from build123d import *

# Parameters (mm, degrees)
SKETCH1_R           = 8
SKETCH1_R_2         = 1.75
BOSS_EXTRUDE1_DEPTH = 6.35
FILLET1_R           = 10


with BuildPart() as part:
    # Sketch1 → Boss-Extrude1 (new body)
    with BuildSketch(Plane(origin=(0, 0, 0), x_dir=(1, 0, 0), z_dir=(0, 1, 0))):
        Polygon((0, 44.633081493), (33.8, 0), (88, 0), (88, 300), (33.8, 300), (0, 280.510901235), align=None)
        with Locations(Location((13, 49, 0), (0, 0, 270))):
            Circle(SKETCH1_R, mode=Mode.SUBTRACT)
        with Locations(Location((38.8, 25, 0), (0, 0, 270))):
            Circle(SKETCH1_R_2, mode=Mode.SUBTRACT)
        with Locations(Location((38.8, 69.2, 0), (0, 0, 270))):
            Circle(SKETCH1_R_2, mode=Mode.SUBTRACT)
        with Locations(Location((18, 84.2, 0), (0, 0, 270))):
            Circle(SKETCH1_R_2, mode=Mode.SUBTRACT)
        with Locations(Location((45, 5, 0), (0, 0, 270))):
            Circle(SKETCH1_R_2, mode=Mode.SUBTRACT)
        with Locations(Location((76.8, 5, 0), (0, 0, 270))):
            Circle(SKETCH1_R_2, mode=Mode.SUBTRACT)
        with Locations(Location((83, 25, 0), (0, 0, 270))):
            Circle(SKETCH1_R_2, mode=Mode.SUBTRACT)
        with Locations(Location((83, 69.2, 0), (0, 0, 270))):
            Circle(SKETCH1_R_2, mode=Mode.SUBTRACT)
        with Locations(Location((70, 84.2, 0), (0, 0, 270))):
            Circle(SKETCH1_R_2, mode=Mode.SUBTRACT)
        with Locations(Location((18, 211.2, 0), (0, 0, 270))):
            Circle(SKETCH1_R_2, mode=Mode.SUBTRACT)
        with Locations(Location((4, 226.2, 0), (0, 0, 270))):
            Circle(SKETCH1_R_2, mode=Mode.SUBTRACT)
        with Locations(Location((4, 278.2, 0), (0, 0, 270))):
            Circle(SKETCH1_R_2, mode=Mode.SUBTRACT)
        with Locations(Location((70, 211.2, 0), (0, 0, 270))):
            Circle(SKETCH1_R_2, mode=Mode.SUBTRACT)
        with Locations(Location((45, 295, 0), (0, 0, 270))):
            Circle(SKETCH1_R_2, mode=Mode.SUBTRACT)
        with Locations(Location((84, 226.2, 0), (0, 0, 270))):
            Circle(SKETCH1_R_2, mode=Mode.SUBTRACT)
        with Locations(Location((76.8, 295, 0), (0, 0, 270))):
            Circle(SKETCH1_R_2, mode=Mode.SUBTRACT)
        with Locations(Location((84, 278.2, 0), (0, 0, 270))):
            Circle(SKETCH1_R_2, mode=Mode.SUBTRACT)
    extrude(amount=BOSS_EXTRUDE1_DEPTH)

    # Fillet1
    fillet1_edges = [part.edges().sort_by_distance(p)[0] for p in [
        (88, 3.175, -300),
        (88, 3.175, 0),
        (33.8, 3.175, 0),
        (0, 3.175, -44.633081493),
        (0, 3.175, -280.510901235),
        (33.8, 3.175, -300),
    ]]
    fillet(fillet1_edges, radius=FILLET1_R)


solid = part.part
Geometry check sheet. Reference: the model listing, model coordinates, mm. Round coordinates to 2 decimals unless told otherwise and drop trailing zeros. Order: outer loops, then holes, each group sorted by start corner. A loop starts at its lowest first (then second) coordinate and runs counter-clockwise, first axis right, second up. Notation, with made-up numbers: M -7.5,22 L 47.5,22 A14 cw 47.5,45 Z; hole C 46,16.5 d4. An arc over 180 degrees is marked long. Answer in a Markdown table with one row per item. Add a question column.
Item 1: Material ranges on L1, parallel to X at y = 4.5, z = -211.2; L2, parallel to Z at x = 70, y = 5; L3, parallel to Z at x = 83, y = 2, recorded low to high. Write a range as [from, to].
Item 2: Draft check along Y on faces 1 (the face through (43, 6.35, -152)), 2 (the face through (43, 0, -152)), 3 (the face through (8.132, 3.131, -55.349)). Enter one of: released by +Y, released by -Y, zero draft, split by the parting line, or undercut.
Item 3: Sectioned sample at B-B, the plane x = 8.5. Enter the section's corners in (y, z), plus the area to 3 significant figures.
Item 4: Sectioned sample at A-A, the plane y = 3. State how many separate pieces and enclosed holes the cut face has, plus the area to 3 significant figures.
Item 5: Depth check by flat-ended pin: pin 1 Ø4 at (x, z) = (83, -25) entering from +Y; pin 2 Ø1 at (x, y) = (10.5, 3) entering from -Z; pin 3 Ø1 at (y, z) = (1.5, -31) entering from -X. Enter the tip coordinate at first touch or a pass-through.
Filled in:
| question | item | result |
|---|---|---|
| 1 | L1 | x = [0, 16.25], [19.75, 68.25], [71.75, 88] |
| 1 | L2 | z = [-300, -212.95], [-209.45, -85.95], [-82.45, 0] |
| 1 | L3 | z = [-298.66, -279.64], [-276.76, -227.64], [-224.76, -70.95], [-67.45, -26.75], [-23.25, -1.34] |
| 2 | face 1 | released by +Y |
| 2 | face 2 | released by -Y |
| 2 | face 3 | zero draft |
| 3 | outline | M 0,-285.41 L 6.35,-285.41 L 6.35,-55.61 L 0,-55.61 Z; M 0,-42.39 L 6.35,-42.39 L 6.35,-33.41 L 0,-33.41 Z |
| 3 | area | 1,520 mm² |
| 4 | separate pieces | 1 |
| 4 | enclosed holes | 17 |
| 4 | area | 24,900 mm² |
| 5 | pin 1 | stops at y = 6.35 |
| 5 | pin 2 | stops at z = -286.85 |
| 5 | pin 3 | stops at x = 9.95 |
